Geometry check sheet. Reference: drawing and pictorial views, mm from the part's lowest x, y, z. A direction names the side the tool comes from. Coordinates: 2 decimals unless noted, no trailing zeros. Write each loop counter-clockwise with the first axis right and the second up, starting at its lowest first coordinate (ties: lowest second). Pieces come first, ordered by that corner, then holes. Notation, with made-up numbers: (31, 3) -> (41, 3) arc R20 ccw to (41, 25) -> close; hole circle Ø7 at (53.25, 4.5). An arc over 180 degrees is marked (long way). Answer in a Markdown table with one row per item.
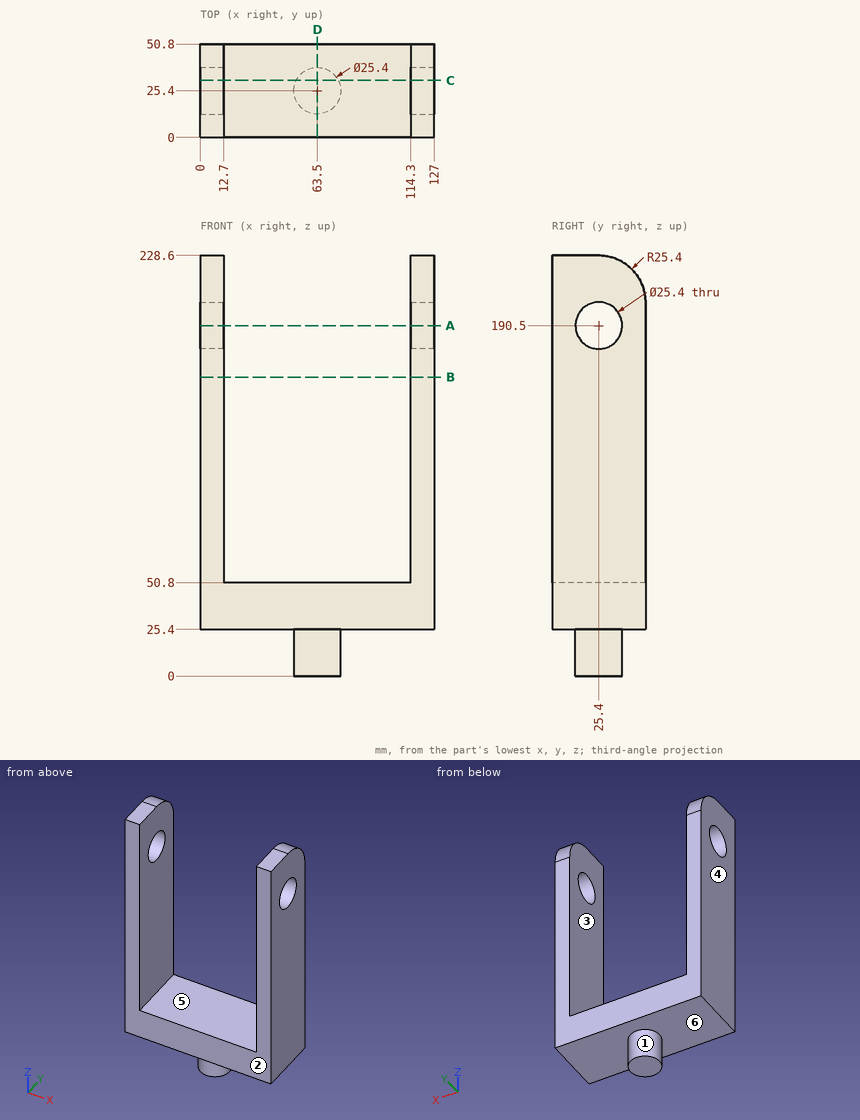
1. Section check A-A, the plane z = 190.5. Record the boundary of the cut face in (x, y).
Geometry says:
| item | result |
|---|---|
| outline | (0, 0) -> (12.7, 0) -> (12.7, 12.7) -> (0, 12.7) -> close; (0, 38.1) -> (12.7, 38.1) -> (12.7, 50.8) -> (0, 50.8) -> close; (114.3, 0) -> (127, 0) -> (127, 12.7) -> (114.3, 12.7) -> close; (114.3, 38.1) -> (127, 38.1) -> (127, 50.8) -> (114.3, 50.8) -> close |
2. Section check D-D, the plane x = 63.5. Record the boundary of the cut face in (y, z).
Geometry says:
| item | result |
|---|---|
| outline | (0, 25.4) -> (12.7, 25.4) -> (12.7, 0) -> (38.1, 0) -> (38.1, 25.4) -> (50.8, 25.4) -> (50.8, 50.8) -> (0, 50.8) -> close |
3. Section check C-C, the plane y = 31. Record the boundary of the cut face in (x, z).
Geometry says:
| item | result |
|---|---|
| outline | (0, 25.4) -> (52.1, 25.4) -> (52.1, 0) -> (74.9, 0) -> (74.9, 25.4) -> (127, 25.4) -> (127, 179.1) -> (114.3, 179.1) -> (114.3, 50.8) -> (12.7, 50.8) -> (12.7, 179.1) -> (0, 179.1) -> close; (0, 201.9) -> (12.7, 201.9) -> (12.7, 227.97) -> (0, 227.97) -> close; (114.3, 201.9) -> (127, 201.9) -> (127, 227.97) -> (114.3, 227.97) -> close |
4. Section check B-B, the plane z = 162.5. Record the boundary of the cut face in (x, y).
Geometry says:
| item | result |
|---|---|
| outline | (0, 0) -> (12.7, 0) -> (12.7, 50.8) -> (0, 50.8) -> close; (114.3, 0) -> (127, 0) -> (127, 50.8) -> (114.3, 50.8) -> close |
5. Mould release check, pull along X, two halves, no side actions. Record for the marked faces 4, 5 and 6: released by +X, released by -X, zero draft, split by the parting line, or undercut.
Geometry says:
| item | result |
|---|---|
| face 4 | released by -X |
| face 5 | undercut |
| face 6 | zero draft |
6. Tool access check on the marked faces 1, 2 and 3. Record the directions out of +Z, -Z, +X, -X, +Y, -Y that give a thin tool (end or side, any length) a straight path to the whole face; none if there is none.
Geometry says:
| item | result |
|---|---|
| face 1 | -Z |
| face 2 | +Z, -Z, +X, -X, -Y |
| face 3 | +Z, +Y, -Y |
7. Depth check by flat-ended pin: P1, Ø6, axis at x = 16, y = 43.5, coming from the +Z side; P2, Ø8, axis at x = 82.5, y = 37, coming from the -Z side. Enter the tip coordinate at first touch or a pass-through.
Geometry says:
| item | result |
|---|---|
| P1 | z = 50.8 |
| P2 | z = 25.4 |
8. Thickness scan on line 1 (X direction, y = 6.5, z = 59.5); line 2 (Y direction, x = 5, z = 190); line 3 (Z direction, x = 117, y = 25). Record the ranges inside material, lowest first. Write a range as from..to.
Geometry says:
| item | result |
|---|---|
| line 1 | 0..12.7, 114.3..127 |
| line 2 | 0..12.71, 38.09..50.8 |
| line 3 | 25.4..177.81, 203.19..228.6 |
